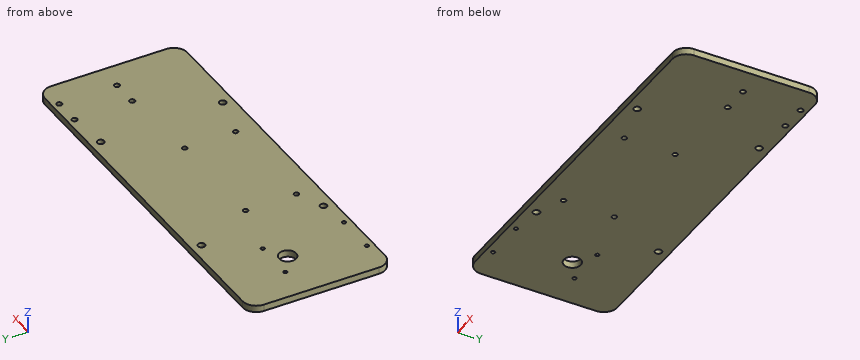
```python
from build123d import *

# Parameters (mm, degrees)
F0_W      = 177.8
F0_H      = 66.675
F1_DEPTH  = 3.175
F3_DEPTH  = 3.176
F5_DEPTH  = 3.176
F6_R      = 1.2573
F7_DEPTH  = 3.176
F8_R      = 1.5875
F9_DEPTH  = 3.176
F10_R     = 0.889
F11_DEPTH = 3.176
F12_R     = 3.9751
F13_DEPTH = 3.176
F14_R     = 1.1303
F15_DEPTH = 3.176


with BuildPart() as f1:
    # F0 (on Top) → F1 (new body)
    with BuildSketch(Plane.XY):
        Rectangle(F0_W, F0_H)
    extrude(amount=F1_DEPTH)

    # F2 (on face) → F3 (cut, through all)
    with BuildSketch(Plane.XY.offset(3.175)):
        with BuildLine():
            ThreePointArc((-88.9, 26.9875), (-87.040128, 31.477628), (-82.55, 33.3375))
            Line((-82.55, 33.3375), (-88.9, 33.3375))
            Line((-88.9, 33.3375), (-88.9, 26.9875))
        make_face()
    extrude(amount=-F3_DEPTH, mode=Mode.SUBTRACT)

    # F4 (on face) → F5 (cut, through all)
    with BuildSketch(Plane.XY.offset(3.175)):
        with BuildLine():
            Line((88.9, 33.3375), (82.55, 33.3375))
            ThreePointArc((82.55, 33.3375), (87.040128, 31.477628), (88.9, 26.9875))
            Line((88.9, 26.9875), (88.9, 33.3375))
        make_face()
        with BuildLine():
            ThreePointArc((88.9, -26.9875), (87.040128, -31.477628), (82.55, -33.3375))
            Line((82.55, -33.3375), (88.9, -33.3375))
            Line((88.9, -33.3375), (88.9, -26.9875))
        make_face()
        with BuildLine():
            ThreePointArc((-82.55, -33.3375), (-87.040128, -31.477628), (-88.9, -26.9875))
            Line((-88.9, -26.9875), (-88.9, -33.3375))
            Line((-88.9, -33.3375), (-82.55, -33.3375))
        make_face()
    extrude(amount=-F5_DEPTH, mode=Mode.SUBTRACT)

    # F6 (on face) → F7 (cut, through all)
    with BuildSketch(Plane.XY.offset(3.175)):
        with Locations((63.5, 30.1625)):
            Circle(F6_R)
        with Locations((76.2, 30.1625)):
            Circle(F6_R)
        with Locations((63.5, 3.1623)):
            Circle(F6_R)
        with Locations((76.2, 3.1623)):
            Circle(F6_R)
    extrude(amount=-F7_DEPTH, mode=Mode.SUBTRACT)

    # F8 (on face) → F9 (cut, through all)
    with BuildSketch(Plane.XY.offset(3.175)):
        with Locations((44.4754, 28.5623)):
            Circle(F8_R)
        with Locations((-39.6748, 28.5623)):
            Circle(F8_R)
        with Locations((-39.6748, -28.5623)):
            Circle(F8_R)
        with Locations((44.4754, -28.5623)):
            Circle(F8_R)
    extrude(amount=-F9_DEPTH, mode=Mode.SUBTRACT)

    # F10 (on face) → F11 (cut, through all)
    with BuildSketch(Plane.XY.offset(3.175)):
        with Locations((-73.025, 7.9375)):
            Circle(F10_R)
        with Locations((-53.975, 7.9375)):
            Circle(F10_R)
        with Locations((-73.025, -30.1625)):
            Circle(F10_R)
        with Locations((-53.975, -30.1625)):
            Circle(F10_R)
    extrude(amount=-F11_DEPTH, mode=Mode.SUBTRACT)

    # F12 (on face) → F13 (cut, through all)
    with BuildSketch(Plane.XY.offset(3.175)):
        with Locations((-63.5, 1.5875)):
            Circle(F12_R)
    extrude(amount=-F13_DEPTH, mode=Mode.SUBTRACT)

    # F14 (on face) → F15 (cut, through all)
    with BuildSketch(Plane.XY.offset(3.175)):
        with Locations((-26.9748, 0.8001)):
            Circle(F14_R)
        with Locations((23.8252, 0.8001)):
            Circle(F14_R)
        with Locations((23.8252, -23.0251)):
            Circle(F14_R)
        with Locations((-26.9748, -23.0251)):
            Circle(F14_R)
    extrude(amount=-F15_DEPTH, mode=Mode.SUBTRACT)


solid = f1.part
```
For this review, take the finished solid that the model builds, in its own axes (mm). Coordinates: 2 decimals unless noted, no trailing zeros. Order: outer loops, then holes, each group sorted by start corner. A loop starts at its lowest first (then second) coordinate and runs counter-clockwise, first axis right, second up. Notation, with made-up numbers: (65, -21) - (117, -21) arc R16 cw to (117, 1) - close; hole circle Ø8 at (-40, 41.5). An arc over 180 degrees is marked (long way). Answer as a JSON object with one key per item and string values. Group by question number.
1. We need section A-A on x = -63.5. State the section outline as (y, z) points (1 decimal).
2. Clearance check with flat-ended pins moving along their axes: P1, Ø3.5, axis at x = 23.83, y = 0.8, coming from the -Z side; P2, Ø1.5, axis at x = 63.5, y = 3.16, coming from the +Z side. State where each tip first meets the part, or that it passes through.
3. For probe 1 along Y at (x, z) = (-28, 2.15); probe 2 along X at (y, z) = (30.5, 2.2); probe 3 along X at (y, z) = (27.5, 0.8), list the stretches that pass through material, from the lowest coordinate up.
Final values:
{
 "1": {"outline": "(-33.3, 0) - (-2.4, 0) - (-2.4, 3.2) - (-33.3, 3.2) - close; (5.6, 0) - (33.3, 0) - (33.3, 3.2) - (5.6, 3.2) - close"},
 "2": {"P1": "z = 0", "P2": "through"},
 "3": {"probe 1": "-33.34 to -23.5, -22.55 to 0.32, 1.28 to 33.34", "probe 2": "-87.84 to 62.29, 64.71 to 74.99, 77.41 to 87.84", "probe 3": "-88.88 to -40.85, -38.5 to 43.3, 45.66 to 88.88"}
}
